Geometry: final body of the model. Coordinates: model frame, mm. A direction names the side the tool comes from. Give positions to 0.01 mm unless a question says otherwise; leave off trailing zeros. Write each loop counter-clockwise with the first axis right and the second up, starting at its lowest first coordinate (ties: lowest second). Pieces come first, ordered by that corner, then holes. Notation, with made-up numbers: M -40,66 L -11,66 A7 ccw -11,70 Z; hole C 41,57 d11. An arc over 180 degrees is marked long. Use a Markdown table: item, result. Add a question column.
(1) Cut plane D-D (x = 98). Output: boundary loops of the cut face in (y, z), plus the area to 3 significant figures.
(2) Cut plane A-A (z = 0). Output: boundary loops of the cut face in (x, y), plus the area to 3 significant figures.
(3) Reachability of faces 1 (the cylindrical face through (3.27, -3.317, -27.605)), 2 (the flat face through (68, -19, 19)), 3 (the flat face through (68, -19, -19)), 4 (the flat face through (15, -3, 20)) from +Z, -Z, +X, -X, +Y, -Y: full face, straight path, thin tool, end or side. Return the list, or none.
(4) Cut plane C-C (z = 26). Output: boundary loops of the cut face in (x, y), plus the area to 3 significant figures.
(5) Material intervals for L1, parallel to X at y = -32, z = 26.5; L2, parallel to Y at x = 45.5, z = -27; L3, parallel to Y at x = 88.5, z = -9, sorted ascending.
(6) Draft query along X for faces 5 (the flat face through (63.5, -36, -27.4)), 6 (the flat face through (77, -23, -2)), 7 (the cylindrical face through (88.346, -33.322, -0.042)), 8 (the cylindrical face through (49.4, -2.03, 19.43)). Return one class per face: released by +X, released by -X, zero draft, split by the parting line, or undercut.
(7) Cut plane B-B (y = -22.5). Output: boundary loops of the cut face in (x, z).
(8) Pin query (flat end, axial travel): pin 1 Ø0.8 at (x, z) = (63.5, -26.5) entering from +Y; pin 2 Ø15 at (x, y) = (78, -13) entering from -Z; pin 3 Ø9 at (x, z) = (89, -2.5) entering from +Y; pin 4 Ø20.5 at (x, y) = (83, -12.5) entering from +Z. Return the tip coordinate at first contact, or that it passes through.
```python
from build123d import *

# Parameters (mm, degrees)
FORME_PRINCIPALE_DEPTH  = 35
ESQUISSE3_W             = 50
ESQUISSE3_H             = 40
VIDEMENT_DEPTH          = 86.399063227
BOSSAGE_CROU_DEPTH      = 4
NERVURE3_REACH          = 119.919
ESQUISSE9_WALL_W        = 277.285093932
ESQUISSE9_WALL_H        = 4
CONG_2_R                = 1
CONG_3_R                = 5
CONG_4_R                = 2
ESQUISSE10_R            = 1
ENL_V_MAT_EXTRU_1_DEPTH = 133.589592352
ESQUISSE11_W            = 1
ESQUISSE11_H            = 40
ENL_V_MAT_EXTRU_2_DEPTH = 117.691902033


with BuildPart() as part:
    # Esquisse1 → Forme principale (new, symmetric)
    with BuildSketch(Plane.XY):
        Polygon((0, -38), (0, 0), (68, 0), (68, -38), (64, -38), (63, -34), (64, -34), (64, -4), (4, -4), (4, -34), (5, -34), (4, -38), align=None)
    extrude(amount=FORME_PRINCIPALE_DEPTH, both=True)

    # Esquisse3 → videment (cut, through all)
    with BuildSketch(Plane(origin=(0, 0, 0), x_dir=(1, 0, 0), z_dir=(0, 1, 0))):
        with Locations((25, 0)):
            Rectangle(ESQUISSE3_W, ESQUISSE3_H)
    extrude(amount=-VIDEMENT_DEPTH, mode=Mode.SUBTRACT)

    # Esquisse4 → Bossage écrou (add)
    with BuildSketch(Plane.XZ.offset(38)):
        with BuildLine():
            Line((68, 15), (99.767786128, 7.802238923))
            ThreePointArc((99.767786128, 7.802238923), (106, 0), (99.767786128, -7.802238923))
            Line((99.767786128, -7.802238923), (68, -15))
            Line((68, -15), (68, 15))
        make_face()
    extrude(amount=-BOSSAGE_CROU_DEPTH)

    # Esquisse7 → Fraisage pour vis à tête fraisée M41 (revolve, cut)
    with BuildSketch(Plane(origin=(98, -34, 0), x_dir=(0, 0, 1), z_dir=(1, 0, 0))):
        Polygon((0, 0), (0, 4.00005), (2.25, 4.00005), (2.25, 2.45), (4.7, 0), align=None)
    revolve(axis=Axis((98, -27.65, 0), (0, -1, 0)), mode=Mode.SUBTRACT)

    # Esquisse9 wall → Nervure3 (add, up to next)
    with BuildSketch(Plane(origin=(78, -17, 0), x_dir=(0.507020126563, -0.861934215158, 0), z_dir=(0.861934215158, 0.507020126563, 0)), mode=Mode.PRIVATE) as nervure3_sk1:
        Rectangle(ESQUISSE9_WALL_W, ESQUISSE9_WALL_H)
    nervure3_tool1 = extrude(nervure3_sk1.sketch, amount=-NERVURE3_REACH, mode=Mode.PRIVATE) - part.part
    add(nervure3_tool1.solids().sort_by_distance((78, -17, 0))[0])

    # Congé2
    cong_2_edges = [part.edges().sort_by_distance(p)[0] for p in [
        (68, -34, -8.5),
        (78, -34, -2),
        (68, -17, -2),
        (78, -34, 2),
        (68, -34, 8.5),
        (68, -17, 2),
        (68, -36, -15),
        (68, -36, 15),
    ]]
    fillet(cong_2_edges, radius=CONG_2_R)

    # Congé3
    cong_3_edges = [part.edges().sort_by_distance(p)[0] for p in [
        (88, -34, 0),
    ]]
    fillet(cong_3_edges, radius=CONG_3_R)

    # Congé4
    cong_4_edges = [part.edges().sort_by_distance(p)[0] for p in [
        (50, -2, -20),
        (50, -2, 20),
    ]]
    fillet(cong_4_edges, radius=CONG_4_R)

    # Esquisse10 → Enlèv. mat.-Extru.1 (cut, through all)
    with BuildSketch(Plane(origin=(0, 0, -35), x_dir=(-1, 0, 0), z_dir=(0, 0, -1))):
        with Locations((-64, -4)):
            Circle(ESQUISSE10_R)
        with Locations((-4, -4)):
            Circle(ESQUISSE10_R)
    extrude(amount=-ENL_V_MAT_EXTRU_1_DEPTH, mode=Mode.SUBTRACT)

    # Esquisse11 → Enlèv. mat.-Extru.2 (cut, through all)
    with BuildSketch(Plane(origin=(0, -34, 0), x_dir=(1, 0, 0), z_dir=(0, 1, 0))):
        with Locations((63.5, 0)):
            Rectangle(ESQUISSE11_W, ESQUISSE11_H)
    extrude(amount=-ENL_V_MAT_EXTRU_2_DEPTH, mode=Mode.SUBTRACT)


solid = part.part
```
Answer list:
| question | item | result |
|---|---|---|
| 1 | outline | M -38,-8.2 L -34,-8.2 L -34,-4.7 L -36.45,-2.25 L -38,-2.25 Z; M -38,2.25 L -36.45,2.25 L -34,4.7 L -34,8.2 L -38,8.2 Z |
| 1 | area | 41.6 mm² |
| 2 | outline | M 50,-4 L 63,-4 A1 cw long 64,-5 L 64,-38 L 95.75,-38 L 95.75,-36.45 L 93.3,-34 L 90.86,-34 A5 cw 86.55,-31.54 L 68,0 L 50,0 Z; M 100.25,-38 L 106,-38 L 106,-34 L 102.7,-34 L 100.25,-36.45 Z |
| 2 | area | 675 mm² |
| 3 | face 1 | +Z, -Z |
| 3 | face 2 | +Z, +X, +Y |
| 3 | face 3 | -Z, +X, +Y |
| 3 | face 4 | -X, +Y, -Y |
| 4 | outline | M 0,-38 L 4,-38 L 5,-34 L 4,-34 L 4,-5 A1 cw long 5,-4 L 63,-4 A1 cw long 64,-5 L 64,-34 L 63,-34 L 64,-38 L 68,-38 L 68,0 L 0,0 Z |
| 4 | area | 543 mm² |
| 5 | L1 | 0 to 4, 64 to 68 |
| 5 | L2 | -4 to 0 |
| 5 | L3 | -38 to -34 |
| 6 | face 5 | undercut |
| 6 | face 6 | zero draft |
| 6 | face 7 | released by +X |
| 6 | face 8 | released by -X |
| 7 | outline | M 0,-35 L 4,-35 L 4,-20 L 0,-20 Z; M 0,20 L 4,20 L 4,35 L 0,35 Z; M 64,-35 L 68,-35 L 68,-3 A1 cw 69,-2 L 81.24,-2 L 81.24,2 L 69,2 A1 cw 68,3 L 68,35 L 64,35 Z |
| 8 | pin 1 | y = 0 |
| 8 | pin 2 | z = -2 |
| 8 | pin 3 | y = -28.1 |
| 8 | pin 4 | z = 2 |
